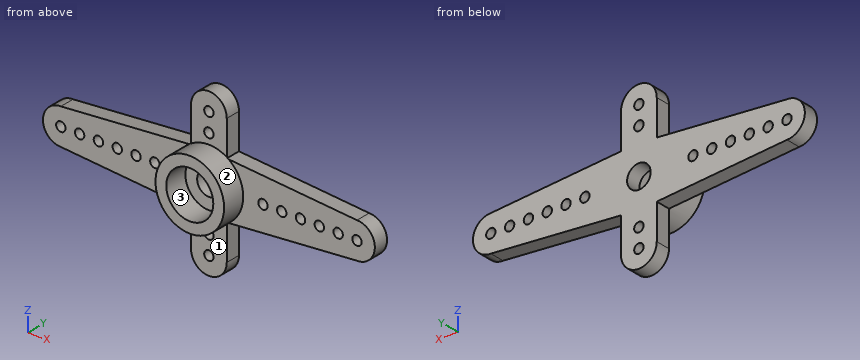
```python
from build123d import *

# Parameters (mm, degrees)
SKETCH1_R           = 3.65
SKETCH1_R_2         = 2.5
BOSS_EXTRUDE1_DEPTH = 2.5
SKETCH2_R           = 1.25
BOSS_EXTRUDE2_DEPTH = 1.6
CUT_EXTRUDE1_REACH  = 6.1
SKETCH3_R           = 0.5


with BuildPart() as part:
    # Sketch1 → Boss-Extrude1 (new body)
    with BuildSketch(Plane(origin=(0, 0, 0), x_dir=(1, 0, 0), z_dir=(0, 1, 0))):
        Circle(SKETCH1_R)
        Circle(SKETCH1_R_2, mode=Mode.SUBTRACT)
    extrude(amount=BOSS_EXTRUDE1_DEPTH)

    # Sketch2 → Boss-Extrude2 (add)
    with BuildSketch(Plane(origin=(0, 2.5, 0), x_dir=(1, 0, 0), z_dir=(0, 1, 0))):
        with BuildLine():
            Line((-1.9, 6.75), (-1.9, 3))
            Line((-1.9, 3), (-15.75, 1.9))
            ThreePointArc((-15.75, 1.9), (-17.65, 0), (-15.75, -1.9))
            Line((-15.75, -1.9), (-1.9, -3))
            Line((-1.9, -3), (-1.9, -6.75))
            ThreePointArc((-1.9, -6.75), (0, -8.65), (1.9, -6.75))
            Line((1.9, -6.75), (1.9, -3))
            Line((1.9, -3), (15.75, -1.9))
            ThreePointArc((15.75, -1.9), (17.65, 0), (15.75, 1.9))
            Line((15.75, 1.9), (1.9, 3))
            Line((1.9, 3), (1.9, 6.75))
            ThreePointArc((1.9, 6.75), (0, 8.65), (-1.9, 6.75))
        make_face()
        Circle(SKETCH2_R, mode=Mode.SUBTRACT)
    extrude(amount=BOSS_EXTRUDE2_DEPTH)

    # Sketch3 → Cut-Extrude1 (cut, up to next)
    with BuildSketch(Plane(origin=(0, 4.1, 0), x_dir=(1, 0, 0), z_dir=(0, 1, 0)), mode=Mode.PRIVATE) as cut_extrude1_sk1:
        with Locations((0, 6.75)):
            Circle(SKETCH3_R)
    cut_extrude1_tool1 = extrude(cut_extrude1_sk1.sketch, amount=-CUT_EXTRUDE1_REACH, mode=Mode.PRIVATE) & part.part
    add(cut_extrude1_tool1.solids().sort_by_distance((0, 4.1, -6.75))[0], mode=Mode.SUBTRACT)
    # Sketch3 → Cut-Extrude1 (cut, up to next)
    with BuildSketch(Plane(origin=(0, 4.1, 0), x_dir=(1, 0, 0), z_dir=(0, 1, 0)), mode=Mode.PRIVATE) as cut_extrude1_sk2:
        with Locations((0, 4.75)):
            Circle(SKETCH3_R)
    cut_extrude1_tool2 = extrude(cut_extrude1_sk2.sketch, amount=-CUT_EXTRUDE1_REACH, mode=Mode.PRIVATE) & part.part
    add(cut_extrude1_tool2.solids().sort_by_distance((0, 4.1, -4.75))[0], mode=Mode.SUBTRACT)
    # Sketch3 → Cut-Extrude1 (cut, up to next)
    with BuildSketch(Plane(origin=(0, 4.1, 0), x_dir=(1, 0, 0), z_dir=(0, 1, 0)), mode=Mode.PRIVATE) as cut_extrude1_sk3:
        with Locations((-15.75, 0)):
            Circle(SKETCH3_R)
    cut_extrude1_tool3 = extrude(cut_extrude1_sk3.sketch, amount=-CUT_EXTRUDE1_REACH, mode=Mode.PRIVATE) & part.part
    add(cut_extrude1_tool3.solids().sort_by_distance((-15.75, 4.1, 0))[0], mode=Mode.SUBTRACT)
    # Sketch3 → Cut-Extrude1 (cut, up to next)
    with BuildSketch(Plane(origin=(0, 4.1, 0), x_dir=(1, 0, 0), z_dir=(0, 1, 0)), mode=Mode.PRIVATE) as cut_extrude1_sk4:
        with Locations((-13.75, 0)):
            Circle(SKETCH3_R)
    cut_extrude1_tool4 = extrude(cut_extrude1_sk4.sketch, amount=-CUT_EXTRUDE1_REACH, mode=Mode.PRIVATE) & part.part
    add(cut_extrude1_tool4.solids().sort_by_distance((-13.75, 4.1, 0))[0], mode=Mode.SUBTRACT)
    # Sketch3 → Cut-Extrude1 (cut, up to next)
    with BuildSketch(Plane(origin=(0, 4.1, 0), x_dir=(1, 0, 0), z_dir=(0, 1, 0)), mode=Mode.PRIVATE) as cut_extrude1_sk5:
        with Locations((-11.75, 0)):
            Circle(SKETCH3_R)
    cut_extrude1_tool5 = extrude(cut_extrude1_sk5.sketch, amount=-CUT_EXTRUDE1_REACH, mode=Mode.PRIVATE) & part.part
    add(cut_extrude1_tool5.solids().sort_by_distance((-11.75, 4.1, 0))[0], mode=Mode.SUBTRACT)
    # Sketch3 → Cut-Extrude1 (cut, up to next)
    with BuildSketch(Plane(origin=(0, 4.1, 0), x_dir=(1, 0, 0), z_dir=(0, 1, 0)), mode=Mode.PRIVATE) as cut_extrude1_sk6:
        with Locations((-9.75, 0)):
            Circle(SKETCH3_R)
    cut_extrude1_tool6 = extrude(cut_extrude1_sk6.sketch, amount=-CUT_EXTRUDE1_REACH, mode=Mode.PRIVATE) & part.part
    add(cut_extrude1_tool6.solids().sort_by_distance((-9.75, 4.1, 0))[0], mode=Mode.SUBTRACT)
    # Sketch3 → Cut-Extrude1 (cut, up to next)
    with BuildSketch(Plane(origin=(0, 4.1, 0), x_dir=(1, 0, 0), z_dir=(0, 1, 0)), mode=Mode.PRIVATE) as cut_extrude1_sk7:
        with Locations((-7.75, 0)):
            Circle(SKETCH3_R)
    cut_extrude1_tool7 = extrude(cut_extrude1_sk7.sketch, amount=-CUT_EXTRUDE1_REACH, mode=Mode.PRIVATE) & part.part
    add(cut_extrude1_tool7.solids().sort_by_distance((-7.75, 4.1, 0))[0], mode=Mode.SUBTRACT)
    # Sketch3 → Cut-Extrude1 (cut, up to next)
    with BuildSketch(Plane(origin=(0, 4.1, 0), x_dir=(1, 0, 0), z_dir=(0, 1, 0)), mode=Mode.PRIVATE) as cut_extrude1_sk8:
        with Locations((-5.75, 0)):
            Circle(SKETCH3_R)
    cut_extrude1_tool8 = extrude(cut_extrude1_sk8.sketch, amount=-CUT_EXTRUDE1_REACH, mode=Mode.PRIVATE) & part.part
    add(cut_extrude1_tool8.solids().sort_by_distance((-5.75, 4.1, 0))[0], mode=Mode.SUBTRACT)
    # Sketch3 → Cut-Extrude1 (cut, up to next)
    with BuildSketch(Plane(origin=(0, 4.1, 0), x_dir=(1, 0, 0), z_dir=(0, 1, 0)), mode=Mode.PRIVATE) as cut_extrude1_sk9:
        with Locations((5.75, 0)):
            Circle(SKETCH3_R)
    cut_extrude1_tool9 = extrude(cut_extrude1_sk9.sketch, amount=-CUT_EXTRUDE1_REACH, mode=Mode.PRIVATE) & part.part
    add(cut_extrude1_tool9.solids().sort_by_distance((5.75, 4.1, 0))[0], mode=Mode.SUBTRACT)
    # Sketch3 → Cut-Extrude1 (cut, up to next)
    with BuildSketch(Plane(origin=(0, 4.1, 0), x_dir=(1, 0, 0), z_dir=(0, 1, 0)), mode=Mode.PRIVATE) as cut_extrude1_sk10:
        with Locations((7.75, 0)):
            Circle(SKETCH3_R)
    cut_extrude1_tool10 = extrude(cut_extrude1_sk10.sketch, amount=-CUT_EXTRUDE1_REACH, mode=Mode.PRIVATE) & part.part
    add(cut_extrude1_tool10.solids().sort_by_distance((7.75, 4.1, 0))[0], mode=Mode.SUBTRACT)
    # Sketch3 → Cut-Extrude1 (cut, up to next)
    with BuildSketch(Plane(origin=(0, 4.1, 0), x_dir=(1, 0, 0), z_dir=(0, 1, 0)), mode=Mode.PRIVATE) as cut_extrude1_sk11:
        with Locations((9.75, 0)):
            Circle(SKETCH3_R)
    cut_extrude1_tool11 = extrude(cut_extrude1_sk11.sketch, amount=-CUT_EXTRUDE1_REACH, mode=Mode.PRIVATE) & part.part
    add(cut_extrude1_tool11.solids().sort_by_distance((9.75, 4.1, 0))[0], mode=Mode.SUBTRACT)
    # Sketch3 → Cut-Extrude1 (cut, up to next)
    with BuildSketch(Plane(origin=(0, 4.1, 0), x_dir=(1, 0, 0), z_dir=(0, 1, 0)), mode=Mode.PRIVATE) as cut_extrude1_sk12:
        with Locations((11.75, 0)):
            Circle(SKETCH3_R)
    cut_extrude1_tool12 = extrude(cut_extrude1_sk12.sketch, amount=-CUT_EXTRUDE1_REACH, mode=Mode.PRIVATE) & part.part
    add(cut_extrude1_tool12.solids().sort_by_distance((11.75, 4.1, 0))[0], mode=Mode.SUBTRACT)
    # Sketch3 → Cut-Extrude1 (cut, up to next)
    with BuildSketch(Plane(origin=(0, 4.1, 0), x_dir=(1, 0, 0), z_dir=(0, 1, 0)), mode=Mode.PRIVATE) as cut_extrude1_sk13:
        with Locations((13.75, 0)):
            Circle(SKETCH3_R)
    cut_extrude1_tool13 = extrude(cut_extrude1_sk13.sketch, amount=-CUT_EXTRUDE1_REACH, mode=Mode.PRIVATE) & part.part
    add(cut_extrude1_tool13.solids().sort_by_distance((13.75, 4.1, 0))[0], mode=Mode.SUBTRACT)
    # Sketch3 → Cut-Extrude1 (cut, up to next)
    with BuildSketch(Plane(origin=(0, 4.1, 0), x_dir=(1, 0, 0), z_dir=(0, 1, 0)), mode=Mode.PRIVATE) as cut_extrude1_sk14:
        with Locations((15.75, 0)):
            Circle(SKETCH3_R)
    cut_extrude1_tool14 = extrude(cut_extrude1_sk14.sketch, amount=-CUT_EXTRUDE1_REACH, mode=Mode.PRIVATE) & part.part
    add(cut_extrude1_tool14.solids().sort_by_distance((15.75, 4.1, 0))[0], mode=Mode.SUBTRACT)
    # Sketch3 → Cut-Extrude1 (cut, up to next)
    with BuildSketch(Plane(origin=(0, 4.1, 0), x_dir=(1, 0, 0), z_dir=(0, 1, 0)), mode=Mode.PRIVATE) as cut_extrude1_sk15:
        with Locations((0, -4.75)):
            Circle(SKETCH3_R)
    cut_extrude1_tool15 = extrude(cut_extrude1_sk15.sketch, amount=-CUT_EXTRUDE1_REACH, mode=Mode.PRIVATE) & part.part
    add(cut_extrude1_tool15.solids().sort_by_distance((0, 4.1, 4.75))[0], mode=Mode.SUBTRACT)
    # Sketch3 → Cut-Extrude1 (cut, up to next)
    with BuildSketch(Plane(origin=(0, 4.1, 0), x_dir=(1, 0, 0), z_dir=(0, 1, 0)), mode=Mode.PRIVATE) as cut_extrude1_sk16:
        with Locations((0, -6.75)):
            Circle(SKETCH3_R)
    cut_extrude1_tool16 = extrude(cut_extrude1_sk16.sketch, amount=-CUT_EXTRUDE1_REACH, mode=Mode.PRIVATE) & part.part
    add(cut_extrude1_tool16.solids().sort_by_distance((0, 4.1, 6.75))[0], mode=Mode.SUBTRACT)


solid = part.part
```
Check sheet for the modelled part. Datum: model origin and axes. Units: mm. Face numbers are marked on the shaded views. Coordinates: 2 decimals unless noted, no trailing zeros. Write each loop counter-clockwise with the first axis right and the second up, starting at its lowest first coordinate (ties: lowest second). Pieces come first, ordered by that corner, then holes. Notation, with made-up numbers: M -29,13.25 L -21,13.25 A9 cw -21,18.25 Z; hole C 57.25,54.25 d11. An arc over 180 degrees is marked long. Write item = value, one per line. Start each with the question number.
1. Sectioned sample at D-D (x = -13.75). Record the cut outline in (y, z).
2. Sectioned sample at B-B (x = 0). State how many separate pieces and enclosed holes the cut face has, then the cut area to 3 significant figures.
3. Mould release check, pull along X, two halves, no side actions. Record for the marked faces 1, 2 and 3: pulls with the +X half, pulls with the -X half, needs draft (parallel to the pull), parting line crosses it, or undercut.
4. Go/stop test with flat-tipped pins: pin 1 (1.8 mm diameter, centred on y = 3.5, z = 5, fed in from +X); pin 2 (3 mm diameter, centred on x = 8.5, z = 2, fed in from -Y); pin 3 (1.8 mm diameter, centred on y = 3.5, z = -5, fed in from -X); pin 4 (6 mm diameter, centred on x = 0, z = 0, fed in from +Y). Record where each tip stops, or that it passes through.
5. Thickness scan on probe 1 along Z at (x, y) = (0, 3); probe 2 along X at (y, z) = (3, -6); probe 3 along Z at (x, y) = (-11.75, 3.5). Record the ranges inside material, lowest first.
6. Sectioned sample at A-A (z = -4.75). Record the cut outline in (x, y).
The answers:
q1.outline = M 2.5,-2.06 L 4.1,-2.06 L 4.1,-0.5 L 2.5,-0.5 Z; M 2.5,0.5 L 4.1,0.5 L 4.1,2.06 L 2.5,2.06 Z
q2.separate_pieces = 6
q2.enclosed_holes = 0
q2.area = 23.0 mm²
q3.face_1 = needs draft
q3.face_2 = parting line crosses it
q3.face_3 = undercut
q4.pin_1 = 1.9
q4.pin_2 = 2.5
q4.pin_3 = -1.9
q4.pin_4 = 4.1
q5.probe_1 = -8.65 to -7.25, -6.25 to -5.25, -4.25 to -1.25, 1.25 to 4.25, 5.25 to 6.25, 7.25 to 8.65
q5.probe_2 = -1.9 to 1.9
q5.probe_3 = -2.22 to -0.5, 0.5 to 2.22
q6.outline = M -1.9,2.5 L -0.5,2.5 L -0.5,4.1 L -1.9,4.1 Z; M 0.5,2.5 L 1.9,2.5 L 1.9,4.1 L 0.5,4.1 Z
